Autodesk Inventor part; units mm, degrees
ref_plane "YZ Plane" through (0, 0, 0) normal (1, 0, 0) x (0, 1, 0)
ref_plane "XZ Plane" through (0, 0, 0) normal (0, 1, 0) x (-1, 0, 0)
ref_plane "XY Plane" through (0, 0, 0) normal (0, 0, 1) x (1, 0, 0)
sketch "Sketch1" plane through (0, 0, 0) normal (0, 0, 1) x (1, 0, 0)
  line L0 (0, 0) -> (533.4, 0)
  line L1 (533.4, 0) -> (533.4, 208.28)
  line L2 (533.4, 208.28) -> (0, 208.28)
  line L3 (0, 208.28) -> (0, 0)
  dimension "d0" = 533.4
  dimension "d1" = 208.28
extrude "Extrusion1" add sketch "Sketch1" along normal blind 12.7
sketch "Sketch2" plane through (0, 0, 12.7) normal (0, 0, 1) x (1, 0, 0)
  line L0 (0, 0) -> (533.4, 0)
  line L1 (355.6, 0) -> (177.8, 0)
  line L2 (177.8, 0) -> (177.8, 165.1)
  line L3 (177.8, 165.1) -> (355.6, 165.1)
  line L4 (355.6, 165.1) -> (355.6, 0)
  line L5 (533.4, 0) -> (533.4, 208.28)
  line L6 (0, 208.28) -> (0, 0)
  dimension "d4" = 165.1
  dimension "d5" = 177.8
  dimension "d6" = 177.8
extrude "Extrusion2" cut sketch "Sketch2" against normal blind 12.7
sketch "Sketch3" plane through (0, 0, 12.7) normal (0, 0, 1) x (1, 0, 0)
  circle A0 centre (423.926, 31.75) radius 4.1656
  line L0 (533.4, 0) -> (533.4, 208.28)
  circle A1 centre (109.474, 31.75) radius 4.1656
  line L1 (0, 208.28) -> (0, 0)
  line L2 (0, 0) -> (177.8, 0)
  line L3 (355.6, 0) -> (533.4, 0)
  dimension "d9" = 109.474
  dimension "d10" = 8.3312
  dimension "d11" = 8.3312
  dimension "d12" = 109.474
  dimension "d13" = 31.75
  dimension "d14" = 31.75
extrude "Extrusion3" cut sketch "Sketch3" against normal blind 25.4
properties part number "Front wall" material "Polycarbonate, Clear"
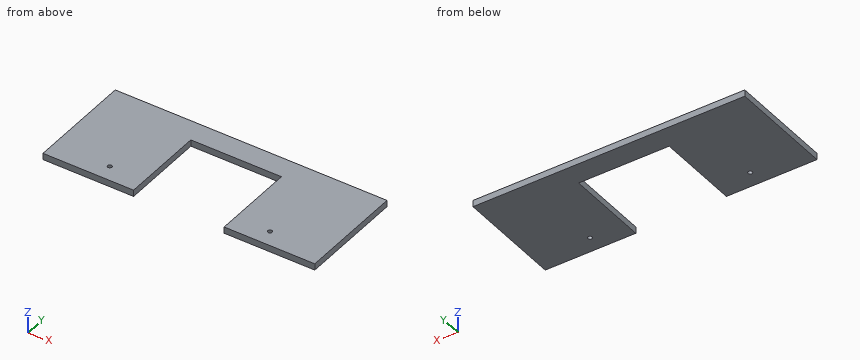
CAD build for the part. Positions are in the model's coordinates, mm. Coordinates: 2 decimals unless noted, no trailing zeros. Order: outer loops, then holes, each group sorted by start corner. A loop starts at its lowest first (then second) coordinate and runs counter-clockwise, first axis right, second up. Notation, with made-up numbers: (-27, 21.5) - (-2, 21.5) arc R8 cw to (-2, 25.5) - close; hole circle Ø9 at (28.25, 70.25). An arc over 180 degrees is marked (long way). Use a Markdown table: item, result. Add a question column.
(1) Saw through at C-C (x = 256). Give the cut face in (y, z).
(2) Saw through at A-A (y = 99). Give the cut face in (x, z), then the cut area to 3 significant figures.
(3) Saw through at B-B (z = 7.75). Give the cut face in (x, y), then the cut area to 3 significant figures.
(4) Drill centre lines: line 1 along X through (y, z) = (162, 3); line 2 along Y through (x, z) = (424.5, 5.25); line 3 along Y through (x, z) = (314, 9.5). Where is each one in solid material? Low to high. Write a range as [from, to].
(5) Flat gauge pin, fed straight in: pin 1 (7.5 mm diameter, centred on x = 109.474, y = 31.75, fed in from +Z). Where does the tip first touch, or does it go through?
Solved:
| question | item | result |
|---|---|---|
| 1 | outline | (165.1, 0) - (208.28, 0) - (208.28, 12.7) - (165.1, 12.7) - close |
| 2 | outline | (0, 0) - (177.8, 0) - (177.8, 12.7) - (0, 12.7) - close; (355.6, 0) - (533.4, 0) - (533.4, 12.7) - (355.6, 12.7) - close |
| 2 | area | 4,520 mm² |
| 3 | outline | (0, 0) - (177.8, 0) - (177.8, 165.1) - (355.6, 165.1) - (355.6, 0) - (533.4, 0) - (533.4, 208.28) - (0, 208.28) - close; hole circle Ø8.33 at (109.47, 31.75); hole circle Ø8.33 at (423.93, 31.75) |
| 3 | area | 81,600 mm² |
| 4 | line 1 | x = [0, 177.8], [355.6, 533.4] |
| 4 | line 2 | y = [0, 27.62], [35.88, 208.28] |
| 4 | line 3 | y = [165.1, 208.28] |
| 5 | pin 1 | passes through |
